from build123d import *

# Parameters (mm, degrees)
SALIENTE_EXTRUIR1_DEPTH = 218
CROQUIS4_W              = 30.00000000000003
CROQUIS4_H              = 96.00000000000001
CROQUIS4_W_2            = 30
CORTAR_EXTRUIR1_DEPTH   = 60
CORTAR_EXTRUIR2_DEPTH   = 10
REDONDEO1_R             = 15


with BuildPart() as part:
    # Croquis2 → Saliente-Extruir1 (new body)
    with BuildSketch(Plane(origin=(0, 0, 0), x_dir=(0, 0, -1), z_dir=(1, 0, 0))):
        Polygon((-60.000000000000014, 35.99999999999998), (-59.99999999999997, -60), (100, -59.99999999999999), align=None)
    extrude(amount=SALIENTE_EXTRUIR1_DEPTH)

    # Croquis3 → Cortar-Recubrir1 section 0
    with BuildSketch(Plane.XY.offset(60)):
        with BuildLine():
            Line((4, 32), (214, 32))
            Line((214, 32), (214, -59.99999999999997))
            Line((214, -59.99999999999997), (4.0000000000000115, -59.99999999999997))
            Line((4.0000000000000115, -59.99999999999997), (4, 32))
        make_face()
    # Croquis3D3 → Cortar-Recubrir1 section 1
    with BuildSketch(Plane(origin=(4, -3.9999999999999964, 0), x_dir=(0.9662349396012463, -0.25766265056033233, 0), z_dir=(0, 0, 1))):
        with BuildLine():
            Line((0, 0), (202.9093373162617, 54.10915661766981))
            Line((202.9093373162617, 54.10915661766981), (217.33844574764032, 0))
            Line((217.33844574764032, 0), (14.42910843137861, -54.1091566176698))
            Line((14.42910843137861, -54.1091566176698), (0, 0))
        make_face()
    loft(mode=Mode.SUBTRACT)

    # Croquis4 → Cortar-Extruir1 (cut)
    with BuildSketch(Plane.XZ.offset(60)):
        Polygon((3.9999999999999982, -4), (33.99999999999999, -4), (34, -100), (4.000000000000011, -100), align=None)
        Polygon((40, -4), (70, -4), (70, -100), (40.000000000000014, -100), align=None)
        Polygon((76.00000000000001, -3.9999999999999973), (106.00000000000001, -3.9999999999999973), (106.00000000000003, -100), (76.00000000000003, -100), align=None)
        Polygon((112.00000000000001, -4), (142.00000000000003, -4), (142.00000000000003, -100), (112.00000000000003, -100), align=None)
        with Locations((199, -52.00000000000001)):
            Rectangle(CROQUIS4_W, CROQUIS4_H)
        with Locations((163.00000000000003, -52.00000000000001)):
            Rectangle(CROQUIS4_W_2, CROQUIS4_H)
    extrude(amount=-CORTAR_EXTRUIR1_DEPTH, mode=Mode.SUBTRACT)

    # Croquis5 → Cortar-Extruir2 (cut)
    with BuildSketch(Plane(origin=(0, 1.7e-16, -3.9999999999999973), x_dir=(-1, 0, 0), z_dir=(0, 4e-17, -1))):
        Polygon((-199, -60), (-184, -60), (-184, -29.999999999999993), (-214.00000000000006, -30), (-214.00000000000003, -60), align=None)
        Polygon((-163.00000000000003, -60), (-148.00000000000003, -60), (-148.00000000000006, -30.000000000000004), (-178.00000000000006, -30.00000000000001), (-178.00000000000006, -60), align=None)
        Polygon((-127, -60), (-112, -60), (-112, -30), (-142.00000000000003, -30.000000000000004), (-142.00000000000003, -60), align=None)
        Polygon((-91.00000000000001, -60), (-76.00000000000001, -59.99999999999999), (-76.00000000000001, -29.999999999999993), (-106.00000000000003, -29.999999999999993), (-106.00000000000001, -60), align=None)
        Polygon((-55.00000000000001, -60), (-40.00000000000001, -60), (-40.00000000000001, -30), (-70.00000000000001, -30.000000000000007), (-70, -60), align=None)
        Polygon((-18.999999999999996, -60), (-3.9999999999999964, -60), (-3.9999999999999964, -30), (-33.99999999999999, -30), (-33.99999999999999, -60), align=None)
    extrude(amount=-CORTAR_EXTRUIR2_DEPTH, mode=Mode.SUBTRACT)

    # Redondeo1
    redondeo1_edges = [part.edges().sort_by_distance(p)[0] for p in [
        (3.9999999999999964, -30, -1.9999999999999993),
        (33.99999999999999, -30, -1.9999999999999991),
        (40.00000000000001, -30, -1.9999999999999993),
        (70.00000000000001, -30.000000000000007, -1.9999999999999993),
        (76.00000000000001, -29.999999999999993, -1.9999999999999991),
        (106.00000000000003, -29.999999999999993, -1.9999999999999993),
        (112, -30, -1.9999999999999993),
        (142.00000000000003, -30.000000000000004, -1.9999999999999993),
        (148.00000000000006, -30.000000000000004, -1.9999999999999993),
        (178.00000000000006, -30.00000000000001, -1.9999999999999993),
        (184, -29.999999999999993, -1.9999999999999993),
        (214.00000000000006, -30, -1.9999999999999993),
    ]]
    fillet(redondeo1_edges, radius=REDONDEO1_R - 0.0001)  # a hair under: the kernel refuses the full size


solid = part.part
Model file for the job. Use its own axes, mm. A direction names the side the tool comes from. Coordinates: 2 decimals unless noted, no trailing zeros. Order: outer loops, then holes, each group sorted by start corner. A loop starts at its lowest first (then second) coordinate and runs counter-clockwise, first axis right, second up. Notation, with made-up numbers: (54.5, -27) -> (97.5, -27) arc R21 cw to (97.5, -16) -> close; hole circle Ø3 at (3.5, 18). An arc over 180 degrees is marked (long way). Return JSON: item names as keys, results as strings. Group by question number.
Item 1: Flat gauge pins, fed straight in: P1, Ø9, axis at x = 61, y = -24.5, coming from the -Z side; P2, Ø5, axis at x = 160, z = -1.5, coming from the +Y side; P3, Ø8, axis at x = 96, y = 18.5, coming from the -Z side; P4, Ø3, axis at x = 97, y = -33.5, coming from the +Z side. Where does each tip first touch, or does it go through?
Item 2: Pull direction X, two halves, no side cores. Call faces 4 (the flat face through (181, -60, -49)), 5 (the flat face through (19, -19, -4)): pulls with the +X half, pulls with the -X half, needs draft (parallel to the pull), parting line crosses it, or undercut.
Item 3: Saw through at D-D on z = 40. Write the cut outline in (x, y).
Item 4: Wall check: line 1 along X through (y, z) = (-13.5, 31); line 2 along Z through (x, y) = (119.5, -19); line 3 along Y through (x, z) = (77, 43.5). Give the ranges that are in metal, low to high. Write a range as [from, to].
Item 5: Saw through at C-C on y = 19.5. Write the cut outline in (x, z), then the cut area to 3 significant figures.
Item 6: Saw through at B-B on z = -72. Write the cut outline in (x, y).
Item 7: Tool access for faces 1 (the flat face through (127, -19, -4)), 2 (the flat face through (109, -60, -49)), 3 (the cylindrical face through (116.51, -34.28, -1.97)): list every direction of +Z, -Z, +X, -X, +Y, -Y with a clear straight run to the whole face (end or side of a thin tool).
Item 8: Saw through at A-A on z = -39. Write the cut outline in (x, y).
Values found:
{
 "1": {"P1": "stops at z = -4", "P2": "stops at y = 0.6", "P3": "stops at z = 24.17", "P4": "passes through"},
 "2": {"face 4": "needs draft", "face 5": "undercut"},
 "3": {"outline": "(0, -60) -> (4, -60) -> (4, 20) -> (214, 20) -> (214, -60) -> (218, -60) -> (218, 24) -> (0, 24) -> close"},
 "4": {"line 1": "x = [0, 4], [214, 218]", "line 2": "z = [-4, 0]", "line 3": "y = [22.1, 26.1]"},
 "5": {"outline": "(0, 32.5) -> (218, 32.5) -> (218, 60) -> (214, 60) -> (214, 39.17) -> (4, 39.17) -> (4, 60) -> (0, 60) -> close", "area": "1,620 mm2"},
 "6": {"outline": "(0, -60) -> (4, -60) -> (4, -43.2) -> (0, -43.2) -> close; (34, -60) -> (40, -60) -> (40, -43.2) -> (34, -43.2) -> close; (70, -60) -> (76, -60) -> (76, -43.2) -> (70, -43.2) -> close; (106, -60) -> (112, -60) -> (112, -43.2) -> (106, -43.2) -> close; (142, -60) -> (148, -60) -> (148, -43.2) -> (142, -43.2) -> close; (178, -60) -> (184, -60) -> (184, -43.2) -> (178, -43.2) -> close; (214, -60) -> (218, -60) -> (218, -43.2) -> (214, -43.2) -> close"},
 "7": {"face 1": "-Z, +Y, -Y", "face 2": "+Z, -Z, +X, -X, -Y", "face 3": "+Z, -Z, -Y"},
 "8": {"outline": "(0, -60) -> (4, -60) -> (4, -23.4) -> (0, -23.4) -> close; (34, -60) -> (40, -60) -> (40, -23.4) -> (34, -23.4) -> close; (70, -60) -> (76, -60) -> (76, -23.4) -> (70, -23.4) -> close; (106, -60) -> (112, -60) -> (112, -23.4) -> (106, -23.4) -> close; (142, -60) -> (148, -60) -> (148, -23.4) -> (142, -23.4) -> close; (178, -60) -> (184, -60) -> (184, -23.4) -> (178, -23.4) -> close; (214, -60) -> (218, -60) -> (218, -23.4) -> (214, -23.4) -> close"}
}
